```python
from build123d import *

# Parameters (mm, degrees)
F0_R      = 126.81364
F1_DEPTH  = 100.688182
F2_R      = 114.205285
F3_DEPTH  = 132.476546
F4_W      = 18.965825
F4_H      = 17.48392
F5_DEPTH  = 25
F7_W      = 34.670085
F7_H      = 27.337872
F7_W_2    = 36.49801
F7_H_2    = 28.232135
F8_DEPTH  = 163.279541
F9_W      = 38.883805
F9_H      = 29.987096
F9_W_2    = 44.849336
F9_W_3    = 36.171764
F10_DEPTH = 212.745748
F11_R     = 127.560498
F12_DEPTH = 14.086724


with BuildPart() as f1:
    # F0 (on Top) → F1 (new body)
    with BuildSketch(Plane.XY):
        Circle(F0_R)
    extrude(amount=F1_DEPTH)

    # F2 (on face) → F3 (cut)
    with BuildSketch(Plane.XY.offset(100.688182)):
        Circle(F2_R)
    extrude(amount=-F3_DEPTH, mode=Mode.SUBTRACT)

    # F7 (on Right) → F8 (cut, symmetric)
    with BuildSketch(Plane.YZ):
        with Locations((-54.778769, 87.475028)):
            Rectangle(F7_W, F7_H)
        with Locations((11.338532, 87.922159)):
            Rectangle(F7_W_2, F7_H_2)
    extrude(amount=F8_DEPTH, both=True, mode=Mode.SUBTRACT)

    # F9 (on Front) → F10 (cut, symmetric)
    with BuildSketch(Plane.XZ):
        with Locations((-67.055523, 90.25082)):
            Rectangle(F9_W, F9_H)
        with Locations((9.9428, 90.25082)):
            Rectangle(F9_W_2, F9_H)
        with Locations((73.962882, 90.25082)):
            Rectangle(F9_W_3, F9_H)
    extrude(amount=F10_DEPTH, both=True, mode=Mode.SUBTRACT)

    # F11 (on face) → F12 (join)
    with BuildSketch(Plane.XY):
        Circle(F11_R)
    extrude(amount=-F12_DEPTH)


with BuildPart() as f5:
    # F4 (on Front) → F5 (new body)
    with BuildSketch(Plane.XZ):
        with Locations((-64.803489, 66.289768)):
            Rectangle(F4_W, F4_H)
    extrude(amount=F5_DEPTH)


solid = f1.part
```
The listing builds one solid part. Answer for the finished solid, in the listing's coordinates (mm). A direction names the side the tool comes from. Give positions to 0.01 mm unless a question says otherwise; leave off trailing zeros. Order: outer loops, then holes, each group sorted by start corner. A loop starts at its lowest first (then second) coordinate and runs counter-clockwise, first axis right, second up. Notation, with made-up numbers: M -25,69.5 L 34,69.5 A21 cw 34,101.5 Z; hole C 15.25,50.5 d10. An arc over 180 degrees is marked long. Put each result on its own line as item: value. Start each with the question number.
Item 1: Flat-ended cylindrical pins translate along their axes: P1, Ø3, axis at y = 69, z = 56.5, coming from the +X side; P2, Ø2, axis at x = 15.5, z = 63.5, coming from the -Y side; P3, Ø1, axis at y = 25, z = 63, coming from the -X side. Find the tip coordinate at first contact, or state that the pin passes through.
Item 2: The part is cut by section C-C, the plane x = 0. Determine the outline of the cut face in (y, z), and give its area (3 significant figures).
Item 3: For a pull along X with two mould halves and no side action, classify faces 1 (the face through (55.877, -107, 88)), 2 (the face through (74, 94, 75.257)), 3 (the face through (44, -111, 100.688)) as +X half, -X half, draft (parallel to the pull), parting line (faces both ways), or undercut.
Item 4: The part is cut by section D-D, the plane y = 79.5. Determine the outline of the cut face in (x, z).
Item 5: Find the intervals of material crossed by line 1 along X through (y, z) = (0, 25); line 2 along Z through (x, y) = (-9.5, -9.5), in increasing order.
Item 6: The part is cut by section B-B, the plane z = 15.5. Determine the outline of the cut face in (x, y), and give its area (3 significant figures).
Item 7: The part is cut by section A-A, the plane y = 0. Determine the outline of the cut face in (x, z).
Item 8: Which of the six approach directions +Z, -Z, +X, -X, +Y, -Y give full straight-line access (tool end or side, diameter ignored) to faces 4 (the face through (92.049, -80, 88)), 5 (the face through (114, -37.444, 87)), 6 (the face through (-120, 11, 73.806))?
Answer key:
1. P1: stops at x = 107.36
1. P2: stops at y = -125.98
1. P3: stops at x = -124.42
2. outline: M -127.56,-14.09 L 127.56,-14.09 L 127.56,0 L 126.81,0 L 126.81,75.26 L 114.21,75.26 L 114.21,0 L -114.21,0 L -114.21,75.26 L -126.81,75.26 L -126.81,0 L -127.56,0 Z
2. area: 5,490 mm²
3. face 1: +X half
3. face 2: undercut
3. face 3: draft
4. outline: M -99.76,-14.09 L 99.76,-14.09 L 99.76,0 L 98.8,0 L 98.8,100.69 L 92.05,100.69 L 92.05,75.26 L 81.99,75.26 L 81.99,0 L -81.99,0 L -81.99,75.26 L -86.5,75.26 L -86.5,100.69 L -98.8,100.69 L -98.8,0 L -99.76,0 Z
5. line 1: x = -126.81 to -114.21, 114.21 to 126.81
5. line 2: z = -14.09 to 0
6. outline: C 0,0 d253.63; hole C 0,0 d228.41
6. area: 9,550 mm²
7. outline: M -127.56,-14.09 L 127.56,-14.09 L 127.56,0 L 126.81,0 L 126.81,73.81 L 114.21,73.81 L 114.21,0 L -114.21,0 L -114.21,73.81 L -126.81,73.81 L -126.81,0 L -127.56,0 Z
8. face 4: +Z, +Y, -Y
8. face 5: +Z, +X, -X, -Y
8. face 6: +Z, +X, -X
